from build123d import *

# Parameters (mm, degrees)
SKETCH1_W           = 27.9908
SKETCH1_H           = 66.2178
BOSS_EXTRUDE1_DEPTH = 6.35
SKETCH4_W           = 49.53
SKETCH4_H           = 6.35
BOSS_EXTRUDE3_DEPTH = 76.2
CUT_EXTRUDE1_DEPTH  = 110.091817223


with BuildPart() as part:
    # Sketch1 → Boss-Extrude1 (new body)
    with BuildSketch(Plane.XY):
        with Locations((13.9954, 33.1089)):
            Rectangle(SKETCH1_W, SKETCH1_H)
    extrude(amount=BOSS_EXTRUDE1_DEPTH)

    # Sketch4 → Boss-Extrude3 (add)
    with BuildSketch(Plane.XY.offset(6.35)):
        with Locations((13.9954, 3.175)):
            Rectangle(SKETCH4_W, SKETCH4_H)
    extrude(amount=BOSS_EXTRUDE3_DEPTH)

    # Sketch5 → Cut-Extrude1 (cut, through all)
    with BuildSketch(Plane(origin=(0, 6.35, 0), x_dir=(1, 0, 0), z_dir=(0, 1, 0))):
        Polygon((-10.7696, -82.55), (13.9954, -55.009603144), (38.7604, -82.55), align=None)
    extrude(amount=-CUT_EXTRUDE1_DEPTH, mode=Mode.SUBTRACT)


solid = part.part
The model under review builds one solid part; all positions refer to its coordinate system, in mm. A direction names the side the tool comes from. Give positions to 0.01 mm unless a question says otherwise; leave off trailing zeros. Order: outer loops, then holes, each group sorted by start corner. A loop starts at its lowest first (then second) coordinate and runs counter-clockwise, first axis right, second up. Notation, with made-up numbers: M 11,-20 L 58,-20 A18 cw 58,7 Z; hole C 43,74.25 d5. An arc over 180 degrees is marked long. One line per question, with ' | ' between items. Start each with the question number.
1) Consider section B-B, the plane x = 10. Give the boundary of the cut face in (y, z), then the cut area to 3 significant figures.
2) Consider section C-C, the plane y = 37. Give the boundary of the cut face in (x, z), then the cut area to 3 significant figures.
3) Mouldability with a two-part tool opening along X and no side actions: class faces 5 (the face through (0, 33, 3)), 6 (the face through (1.44, 3.22, 68.97)), 7 (the face through (14, 37, 6.35)) as pulls with the +X half, pulls with the -X half, needs draft (parallel to the pull), parting line crosses it, or undercut.
4) Consider section A-A, the plane z = 63.5. Give the boundary of the cut face in (x, y).
5) For faces 1 (the face through (-5, 3, 6.35)), 2 (the face through (33, 3, 6.35)), 3 (the face through (26.205, 3.219, 68.587)), 4 (the face through (14, 6.35, 35)), list the 3-axis set-ups (+Z, -Z, +X, -X, +Y, -Y) from which the entire face can be reached by the end or side of a thin tool; tool diameter is ignored.
6) Wall thickness on L1, parallel to Y at x = 33.5, z = 69.5; L2, parallel to X at y = 51, z = 5.5: over which ranges is each line inside the solid? List them lowest first. Write a range as from..to.
7) Clearance check with flat-ended pins moving along their axes: P1, Ø22.5, axis at x = 9, y = 23.5, coming from the +Z side; P2, Ø8, axis at x = 23.5, z = 38, coming from the +Y side; P3, Ø5, axis at x = -6.5, y = 3.5, coming from the -Z side. State where each tip first meets the part, or that it passes through.
8) Consider section D-D, the plane z = 26. Give the boundary of the cut face in (x, y).
Found:
1) outline: M 0,0 L 66.22,0 L 66.22,6.35 L 6.35,6.35 L 6.35,59.45 L 0,59.45 Z | area: 758 mm²
2) outline: M 0,0 L 27.99,0 L 27.99,6.35 L 0,6.35 Z | area: 178 mm²
3) face 5: pulls with the -X half | face 6: undercut | face 7: needs draft
4) outline: M -10.77,0 L 6.36,0 L 6.36,6.35 L -10.77,6.35 Z; M 21.63,0 L 38.76,0 L 38.76,6.35 L 21.63,6.35 Z
5) face 1: -Z, -X, +Y, -Y | face 2: -Z, +X, +Y, -Y | face 3: +Z, +Y, -Y | face 4: +Z, +X, -X, +Y
6) L1: y = 0..6.35 | L2: x = 0..27.99
7) P1: stops at z = 6.35 | P2: stops at y = 6.35 | P3: stops at z = 6.35
8) outline: M -10.77,0 L 38.76,0 L 38.76,6.35 L -10.77,6.35 Z
